from build123d import *

# Parameters (mm, degrees)
F1_DEPTH = 10
F2_R     = 2
F3_DEPTH = 4.001
F5_DEPTH = 3
F7_DEPTH = 3
F8_DEPTH = 25


with BuildPart() as f1:
    # F0 (on Top) → F1 (new body)
    with BuildSketch(Plane.XY):
        with BuildLine():
            ThreePointArc((-58.60368, -38.875302), (-43.20368, -23.475302), (-27.80368, -38.875302))
            Line((-27.80368, -38.875302), (-11.80368, -38.875302))
            Line((-11.80368, -38.875302), (-11.80368, -34.875302))
            Line((-11.80368, -34.875302), (-22.662015, -34.875302))
            ThreePointArc((-22.662015, -34.875302), (-23.861703, -34.475536), (-24.581796, -33.43605))
            ThreePointArc((-24.581796, -33.43605), (-43.20368, -19.475302), (-61.825563, -33.43605))
            ThreePointArc((-61.825563, -33.43605), (-62.545656, -34.475536), (-63.745345, -34.875302))
            Line((-63.745345, -34.875302), (-74.60368, -34.875302))
            Line((-74.60368, -34.875302), (-74.60368, -38.875302))
            Line((-74.60368, -38.875302), (-62.60368, -38.875302))
            Line((-62.60368, -38.875302), (-58.60368, -38.875302))
        make_face()
    extrude(amount=F1_DEPTH)

    # F2 (on face) → F3 (cut, through all)
    with BuildSketch(Plane(origin=(0, -34.875302, 0), x_dir=(-1, 0, 0), z_dir=(0, 1, 0))):
        with Locations((69.174512, 5)):
            Circle(F2_R)
        with Locations((19.30368, 5)):
            Circle(F2_R)
    extrude(amount=-F3_DEPTH, mode=Mode.SUBTRACT)

    # F4 (on face) → F5 (cut)
    with BuildSketch(Plane(origin=(0, -34.875302, 0), x_dir=(-1, 0, 0), z_dir=(0, 1, 0))):
        Polygon((65.13306, 5), (67.153786, 1.5), (71.195238, 1.5), (73.215964, 5), (71.195238, 8.5), (67.153786, 8.5), align=None)
    extrude(amount=-F5_DEPTH, mode=Mode.SUBTRACT)

    # F6 (on face) → F7 (cut)
    with BuildSketch(Plane(origin=(0, -34.875302, 0), x_dir=(-1, 0, 0), z_dir=(0, 1, 0))):
        Polygon((15.262228, 5), (17.282954, 1.5), (21.324406, 1.5), (23.345132, 5), (21.324406, 8.5), (17.282954, 8.5), align=None)
    extrude(amount=-F7_DEPTH, mode=Mode.SUBTRACT)

    # F6 (on face) → F8 (cut)
    with BuildSketch(Plane(origin=(0, -34.875302, 0), x_dir=(-1, 0, 0), z_dir=(0, 1, 0))):
        Polygon((15.262228, 5), (17.282954, 1.5), (21.324406, 1.5), (23.345132, 5), (21.324406, 8.5), (17.282954, 8.5), align=None)
    extrude(amount=F8_DEPTH, mode=Mode.SUBTRACT)


solid = f1.part
CAD build for the part. Positions are in the model's coordinates, mm. A direction names the side the tool comes from. Give positions to 0.01 mm unless a question says otherwise; leave off trailing zeros. Loops run counter-clockwise (first coordinate to the right, second up) from the corner with the lowest first, then second, coordinate; pieces in that order, holes last. Notation, with made-up numbers: M 31,14.5 L 70,14.5 A24 ccw 70,33.5 Z; hole C 6,20.5 d8. An arc over 180 degrees is marked long. Write each question's results on one line, items separated by ' | '.
Q1. Probe probe 1 along Y at (x, z) = (-22.5, 1.5); probe 2 along X at (y, z) = (-27, 2); probe 3 along Y at (x, z) = (-43, 7.25). List the from-to ranges inside material, lowest first.
Geometry check:
probe 1: y = -38.88 to -34.88 | probe 2: x = -58.54 to -53.01, -33.4 to -27.86 | probe 3: y = -23.48 to -19.48
Q2. Band-saw the part on B-B on x = -20.5. Write the cut outline in (y, z), and give its area (3 significant figures).
Geometry check:
outline: M -38.88,0 L -34.88,0 L -34.88,1.5 L -37.88,1.5 L -37.88,3.4 L -38.88,3.4 Z; M -38.88,6.6 L -37.88,6.6 L -37.88,8.5 L -34.88,8.5 L -34.88,10 L -38.88,10 Z | area: 15.8 mm²
Q3. Which spindle directions (+Z, -Z, +X, -X, +Y, -Y) get a long thin tool onto all of the face, cutting with end or side? Do faces 5 (the face through (-17.306, -38.368, 5.088)), 6 (the face through (-21, -37.875, 7)). Say none if no direction does.
Geometry check:
face 5: +Y, -Y | face 6: +Y
Q4. Band-saw the part on A-A on y = -31. Write the cut outline in (x, z).
Geometry check:
outline: M -60.93,0 L -56.44,0 L -56.44,10 L -60.93,10 Z; M -29.97,0 L -25.47,0 L -25.47,10 L -29.97,10 Z
Q5. Mould opens along Z. For faces 1 (the face through (-67.176, -38.368, 5.088)), 2 (the face through (-46, -23, 0)), 3 (the face through (-22.349, -36.293, 6.725)), 4 (the face through (-42.85, -19.48, 4.93)) say: pulls with the +Z half, pulls with the -Z half, needs draft (parallel to the pull), parting line crosses it, or undercut.
Geometry check:
face 1: undercut | face 2: pulls with the -Z half | face 3: undercut | face 4: needs draft
Q6. Band-saw the part on C-C on x = -64.5. Write the cut outline in (y, z), and give its area (3 significant figures).
Geometry check:
outline: M -38.88,0 L -34.88,0 L -34.88,10 L -38.88,10 Z | area: 40.0 mm²
Q7. Band-saw the part on D-D on x = -53.5. Write the cut outline in (y, z).
Geometry check:
outline: M -27.42,0 L -22.43,0 L -22.43,10 L -27.42,10 Z
Q8. Flat gauge pins, fed straight in: P1, Ø6, axis at y = -30.5, z = 5.5, coming from the +X side; P2, Ø3, axis at x = -48, z = 1.5, coming from the -Y side; P3, Ø2.5, axis at x = -19.3, z = 5, coming from the -Y side; P4, Ø5, axis at x = -69.17, z = 5, coming from the +Y side. Where does each tip first touch, or does it go through?
Geometry check:
P1: stops at x = -24.56 | P2: stops at y = -24.82 | P3: passes through | P4: stops at y = -37.88
